from build123d import *

# Parameters (mm, degrees)
CUT_EXTRUDE1_REACH      = 29.857
CUT_EXTRUDE1_END_RADIUS = 7.5
SKETCH2_R               = 1.6
CUT_EXTRUDE2_REACH      = 29.857
CUT_EXTRUDE2_END_RADIUS = 7.5
SKETCH3_R               = 1.6


with BuildPart() as part:
    # Sketch1 → Revolve1 (revolve)
    with BuildSketch(Plane.XY, mode=Mode.PRIVATE) as revolve1_sk:
        Polygon((-3.175, 10), (-3.175, 24), (-10, 24), (-10, 23), (-7.5, 23), (-7.5, 11), (-10, 11), (-10, 10), align=None)
    revolve(revolve1_sk.sketch.rotate(Axis((0, 0, 0), (0, 1, 0)), 270), axis=Axis((0, 0, 0), (0, 1, 0)))

    # Cut-Extrude1: up to this cylinder (the profile starts inside it)
    cut_extrude1_end = Plane(origin=(0, 17, 0), z_dir=(0, -1, 0)) * Cylinder(CUT_EXTRUDE1_END_RADIUS, 75.714, mode=Mode.PRIVATE)
    # Sketch2 → Cut-Extrude1 (cut, up to the surface)
    with BuildSketch(Plane.XY, mode=Mode.PRIVATE) as cut_extrude1_sk1:
        with Locations((0, 17)):
            Circle(SKETCH2_R)
    cut_extrude1_tool1 = extrude(cut_extrude1_sk1.sketch, amount=-CUT_EXTRUDE1_REACH, mode=Mode.PRIVATE) & cut_extrude1_end
    add(cut_extrude1_tool1.solids().sort_by_distance((0, 17, 0))[0], mode=Mode.SUBTRACT)

    # Cut-Extrude2: up to this cylinder (the profile starts inside it)
    cut_extrude2_end = Plane(origin=(0, 17, 0), z_dir=(0, -1, 0)) * Cylinder(CUT_EXTRUDE2_END_RADIUS, 75.714, mode=Mode.PRIVATE)
    # Sketch3 → Cut-Extrude2 (cut, up to the surface)
    with BuildSketch(Plane(origin=(0, 0, 0), x_dir=(0, 0, -1), z_dir=(1, 0, 0)), mode=Mode.PRIVATE) as cut_extrude2_sk1:
        with Locations((0, 17)):
            Circle(SKETCH3_R)
    cut_extrude2_tool1 = extrude(cut_extrude2_sk1.sketch, amount=-CUT_EXTRUDE2_REACH, mode=Mode.PRIVATE) & cut_extrude2_end
    add(cut_extrude2_tool1.solids().sort_by_distance((0, 17, 0))[0], mode=Mode.SUBTRACT)


solid = part.part
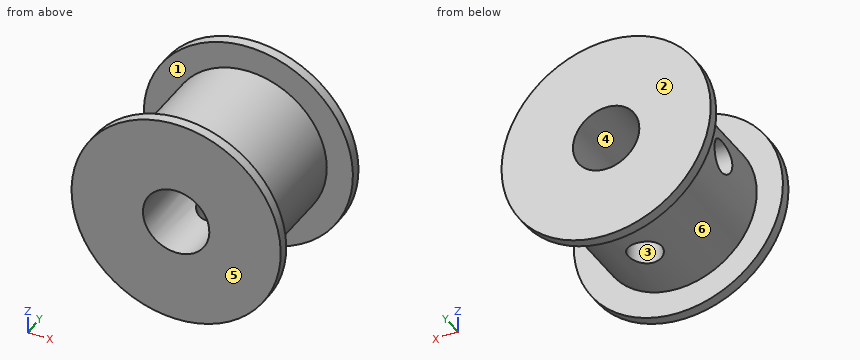
The listing builds one solid part. Answer for the finished solid, in the listing's coordinates (mm). Face numbers are marked on the shaded views. A direction names the side the tool comes from. Give positions to 0.01 mm unless a question says otherwise; leave off trailing zeros. Write each loop counter-clockwise with the first axis right and the second up, starting at its lowest first coordinate (ties: lowest second). Pieces come first, ordered by that corner, then holes. Notation, with made-up numbers: (0, 10.5) -> (36, 10.5) arc R13 ccw to (36, 30.5) -> close; hole circle Ø6 at (-24, 30). An arc over 180 degrees is marked (long way). One line per question, with ' | ' between items. Start each with the question number.
1. Section B-B (z = 0) is taken. Determine the outline of the cut face in (x, y) (3 decimals).
2. Section A-A (x = 0) is taken. Determine the outline of the cut face in (y, z) (3 decimals).
3. Section D-D (y = 17) is taken. Determine the outline of the cut face in (x, z) (3 decimals), plus the area to 3 significant figures.
4. For a pull along Y with two mould halves and no side action, classify the marked faces 4, 5 and 6 as pulls with the +Y half, pulls with the -Y half, needs draft (parallel to the pull), parting line crosses it, or undercut.
5. Find the intervals of material crossed by probe 1 along Y at (x, z) = (7.5, -1); probe 2 along Y at (x, z) = (-5.8, 0); probe 3 along X at (y, z) = (19, 0) (3 decimals), in increasing order.
6. Section C-C (z = -6) is taken. Determine the outline of the cut face in (x, y).
7. For the marked faces 1, 2 and 3, determine the directions among +Z, -Z, +X, -X, +Y, -Y from which every point of the face is accessible in a straight line to the end or side of a thin tool.
8. Given pin 1 Ø5 at (y, z) = (17, 0) entering from +X; pin 2 Ø1 at (y, z) = (15.5, 6.5) entering from -X; pin 3 Ø3 at (x, y) = (0, 19.5) entering from +Z, each flat-ended and moving along its own axis, determine where each tip first touches the part or whether it passes through.
Response values:
1) outline: (-10, 10) -> (-3.175, 10) -> (-3.175, 15.4) -> (-7.5, 15.4) -> (-7.5, 11) -> (-10, 11) -> close; (-10, 23) -> (-7.5, 23) -> (-7.5, 18.6) -> (-3.175, 18.6) -> (-3.175, 24) -> (-10, 24) -> close; (3.175, 10) -> (10, 10) -> (10, 11) -> (7.5, 11) -> (7.5, 23) -> (10, 23) -> (10, 24) -> (3.175, 24) -> close
2) outline: (10, -10) -> (11, -10) -> (11, -7.5) -> (15.4, -7.5) -> (15.4, -3.175) -> (10, -3.175) -> close; (10, 3.175) -> (24, 3.175) -> (24, 10) -> (23, 10) -> (23, 7.5) -> (11, 7.5) -> (11, 10) -> (10, 10) -> close; (18.6, -7.5) -> (23, -7.5) -> (23, -10) -> (24, -10) -> (24, -3.175) -> (18.6, -3.175) -> close
3) outline: (-7.327, -1.6) arc R7.5 ccw to (-1.6, -7.327) -> (-1.6, -2.742) arc R3.175 cw to (-2.742, -1.6) -> close; (-7.327, 1.6) -> (-2.742, 1.6) arc R3.175 cw (long way) to (1.6, -2.742) -> (1.6, -7.327) arc R7.5 ccw (long way) to start | area: 117 mm2
4) face 4: needs draft | face 5: pulls with the -Y half | face 6: undercut
5) probe 1: 10 to 11, 23 to 24 | probe 2: 10 to 15.4, 18.6 to 24 | probe 3: -7.5 to -3.175, 3.175 to 7.5
6) outline: (-8, 10) -> (8, 10) -> (8, 11) -> (4.5, 11) -> (4.5, 23) -> (8, 23) -> (8, 24) -> (-8, 24) -> (-8, 23) -> (-4.5, 23) -> (-4.5, 11) -> (-8, 11) -> close; hole circle Ø3.2 at (0, 17)
7) face 1: none | face 2: +Z, -Z, +X, -X, +Y | face 3: -Z
8) pin 1: x = 7.5 | pin 2: x = -4.5 | pin 3: z = 7.5
